from build123d import *

# Parameters (mm, degrees)
BOSS_EXTRUDE1_DEPTH      = 11.938
BOSS_EXTRUDE1_DEPTH_BACK = 11.938
SKETCH1_W                = 31.75
SKETCH1_H                = 50.8
CUT_EXTRUDE2_DEPTH       = 62.083699495
CUT_EXTRUDE2_DEPTH_BACK  = 3.175
SKETCH3_R                = 1.7272
SKETCH4_R                = 6.35
CUT_EXTRUDE3_DEPTH       = 38.1


with BuildPart() as part:
    # Sketch1 → Boss-Extrude1 (new, two sides: drawn at the far end of the back side and taken through both)
    with BuildSketch(Plane(origin=(0, 0, 0), x_dir=(0, 0, -1), z_dir=(1, 0, 0)).offset(-BOSS_EXTRUDE1_DEPTH_BACK)):
        with Locations((0, -25.4)):
            Rectangle(SKETCH1_W, SKETCH1_H)
    extrude(amount=BOSS_EXTRUDE1_DEPTH + BOSS_EXTRUDE1_DEPTH_BACK)

    # Sketch3 → Cut-Extrude2 (cut, two sides: drawn at the far end of the back side and taken through both)
    with BuildSketch(Plane.XY.offset(15.875).offset(-CUT_EXTRUDE2_DEPTH_BACK)):
        with Locations(Location((7.9375, -19.05, 0), (0, 0, 180))):
            Circle(SKETCH3_R)
        with Locations(Location((-7.9375, -39.6748, 0), (0, 0, 180))):
            Circle(SKETCH3_R)
    extrude(amount=CUT_EXTRUDE2_DEPTH + CUT_EXTRUDE2_DEPTH_BACK, mode=Mode.SUBTRACT)

    # Sketch4 → Cut-Extrude3 (cut)
    with BuildSketch(Plane(origin=(0, 0, 0), x_dir=(1, 0, 0), z_dir=(0, 1, 0))):
        with Locations(Location((0, 0, 0), (0, 0, 270))):
            Circle(SKETCH4_R)
    extrude(amount=-CUT_EXTRUDE3_DEPTH, mode=Mode.SUBTRACT)


solid = part.part
Read the model definition and answer for the solid it produces. Units are mm, in the model's axes. A direction names the side the tool comes from. Round coordinates to 2 decimals unless told otherwise and drop trailing zeros. Write each loop counter-clockwise with the first axis right and the second up, starting at its lowest first coordinate (ties: lowest second). Pieces come first, ordered by that corner, then holes. Notation, with made-up numbers: (-5.75, 16.5) - (1.25, 16.5) arc R29 cw to (1.25, 40.5) - close; hole circle Ø9 at (86, 54.25). An arc over 180 degrees is marked (long way). One line per question, with ' | ' between items. Start each with the question number.
1. This flat-tipped pin is pushed along its axis until it touches: pin 1 (1 mm diameter, centred on x = 8, y = -20, fed in from +Z). Where does it stop, or does it pass through?
2. Find the intervals of material crossed by probe 1 along X at (y, z) = (-27, 0); probe 2 along X at (y, z) = (-19.05, 14); probe 3 along Z at (x, y) = (1.75, -7) (3 decimals), in increasing order. Write a range as [from, to].
3. Section D-D (z = 14) is taken. Determine the outline of the cut face in (x, y), and give its area (3 significant figures).
4. Section A-A (y = -19.05) is taken. Determine the outline of the cut face in (x, z) (3 decimals), and give its area (3 significant figures).
5. For a pull along X with two mould halves and no side action, classify faces 1 (the face through (11.938, -25, 0)), 2 (the face through (0, -50.8, 0)), 3 (the face through (-8, -40, 12.7)) as +X half, -X half, draft (parallel to the pull), parting line (faces both ways), or undercut.
6. For faces 4 (the face through (0, -26, 15.875)), 5 (the face through (8, -19, 12.7)), 6 (the face through (0, -38.1, 0)), determine the directions among +Z, -Z, +X, -X, +Y, -Y from which every point of the face is accessible in a straight line to the end or side of a thin tool.
7. Section B-B (z = 0) is taken. Determine the outline of the cut face in (x, y), and give its area (3 significant figures).
8. Section C-C (x = 0) is taken. Determine the outline of the cut face in (y, z) (3 decimals), and give its area (3 significant figures).
Filled in:
1) pin 1: z = 12.7
2) probe 1: [-11.94, -6.35], [6.35, 11.94] | probe 2: [-11.94, 6.21], [9.66, 11.94] | probe 3: [-15.875, -6.104], [6.104, 15.875]
3) outline: (-11.94, -50.8) - (11.94, -50.8) - (11.94, 0) - (-11.94, 0) - close; hole circle Ø3.45 at (-7.94, -39.67); hole circle Ø3.45 at (7.94, -19.05) | area: 1,190 mm²
4) outline: (-11.938, -15.875) - (11.938, -15.875) - (11.938, 15.875) - (9.665, 15.875) - (9.665, 12.7) - (6.21, 12.7) - (6.21, 15.875) - (-11.938, 15.875) - close; hole circle Ø12.7 at (0, 0) | area: 620 mm²
5) face 1: +X half | face 2: draft | face 3: undercut
6) face 4: +Z, +X, -X, +Y, -Y | face 5: +Z | face 6: +Y
7) outline: (-11.94, -50.8) - (11.94, -50.8) - (11.94, 0) - (6.35, 0) - (6.35, -38.1) - (-6.35, -38.1) - (-6.35, 0) - (-11.94, 0) - close | area: 729 mm²
8) outline: (-50.8, -15.875) - (0, -15.875) - (0, -6.35) - (-38.1, -6.35) - (-38.1, 6.35) - (0, 6.35) - (0, 15.875) - (-50.8, 15.875) - close | area: 1,130 mm²
